Part model, mm, in its own coordinate system. A direction names the side the tool comes from. Give positions to 0.01 mm unless a question says otherwise; leave off trailing zeros. Order: outer loops, then holes, each group sorted by start corner. A loop starts at its lowest first (then second) coordinate and runs counter-clockwise, first axis right, second up. Notation, with made-up numbers: (86.25, 86) -> (107.25, 86) arc R21 ccw to (107.25, 115) -> close; hole circle Ø6 at (15, -15). An arc over 180 degrees is marked (long way). Write item = value, one per line. Start each with the question number.
(1) Probe line 1 along Y through (x, z) = (0, 4.25); line 2 along X through (y, z) = (-3, 4.75); line 3 along Z through (x, y) = (4, 3.25). List the from-to ranges inside material, lowest first. Write a range as from..to.
(2) Two-plate mould, pull along X, no slides. Class faces 3 (the flat face through (0, 0, 0)), 4 (the cylindrical face through (-5.75, 5.27, 6.42)), 5 (the cylindrical face through (8.394, 2.643, 5.916)): pulls with the +X half, pulls with the -X half, needs draft (parallel to the pull), parting line crosses it, or undercut.
(3) Flat gauge pins, fed straight in: pin 1 (6 mm diameter, centred on y = -4.5, z = 2.5, fed in from +X); pin 2 (1.5 mm diameter, centred on x = 6, z = 5, fed in from -Y); pin 3 (6 mm diameter, centred on y = 3.5, z = 8, fed in from -X). Where does each tip first touch, or does it go through?
(4) Saw through at A-A, the plane z = 9. List the corners of the cut face in (x, y), then the cut area to 3 significant figures.
(5) Which spindle directions (+Z, -Z, +X, -X, +Y, -Y) get a long thin tool onto all of the face, cutting with end or side? Do faces 1 (the flat face through (-1, -8, 12)), 2 (the flat face through (0, 0, 1)). Say none if no direction does.
(6) Saw through at B-B, the plane y = 0. List the corners of the cut face in (x, z), then the cut area to 3 significant figures.
from build123d import *

# Parameters (mm, degrees)
CYLINDER002_R     = 7.8
CYLINDER002_DEPTH = 12
CYLINDER003_R     = 8.8
CYLINDER003_DEPTH = 12


with BuildPart() as cylinder002:
    # Cylinder002 → Cylinder002 (new body)
    with BuildSketch(Plane.XY.offset(1)):
        Circle(CYLINDER002_R)
    extrude(amount=CYLINDER002_DEPTH)


with BuildPart() as cut:
    # Cylinder003 → Cylinder003 (new body)
    with BuildSketch(Plane.XY):
        Circle(CYLINDER003_R)
    extrude(amount=CYLINDER003_DEPTH)

    # Cut: cut Cylinder002
    add(cylinder002.part, mode=Mode.SUBTRACT)


solid = cut.part
Results list:
q1.line_1 = -8.8..-7.8, 7.8..8.8
q1.line_2 = -8.27..-7.2, 7.2..8.27
q1.line_3 = 0..1
q2.face_3 = needs draft
q2.face_4 = undercut
q2.face_5 = parting line crosses it
q3.pin_1 = 8.67
q3.pin_2 = -7.06
q3.pin_3 = -8.79
q4.outline = circle Ø17.6 at (0, 0); hole circle Ø15.6 at (0, 0)
q4.area = 52.2 mm^2
q5.face_1 = +Z, +X, -X, +Y, -Y
q5.face_2 = +Z
q6.outline = (-8.8, 0) -> (8.8, 0) -> (8.8, 12) -> (7.8, 12) -> (7.8, 1) -> (-7.8, 1) -> (-7.8, 12) -> (-8.8, 12) -> close
q6.area = 39.6 mm^2
